Autodesk Inventor part; units mm, degrees
ref_plane "YZ Plane" through (0, 0, 0) normal (1, 0, 0) x (0, 1, 0)
ref_plane "XZ Plane" through (0, 0, 0) normal (0, 1, 0) x (-1, 0, 0)
ref_plane "XY Plane" through (0, 0, 0) normal (0, 0, 1) x (1, 0, 0)
sketch "Sketch1" plane through (0, 0, 0) normal (0, 0, 1) x (1, 0, 0)
  line L0 (10, 0) -> (10, 2)
  arc A0 (10, 2) -> (8.5, 3.5) centre (8.5, 2) ccw
  line L1 (8.5, 3.5) -> (-8.5, 3.5)
  arc A1 (-8.5, 3.5) -> (-10, 2) centre (-8.5, 2) ccw
  line L2 (-10, 2) -> (-8, 2)
  line L3 (-8, 2) -> (-8, 0)
  line L4 (-6, 0) -> (-8, 0)
  arc A2 (0, 0) -> (-6, 0) centre (-3, 0) ccw
  line L5 (7, 0) -> (0, 0)
  line L6 (7, 0) -> (7, 2.5)
  line L7 (7, 2.5) -> (9, 2.5)
  line L8 (9, 2.5) -> (9, 0)
  line L9 (10, 0) -> (9, 0)
  line L10 (-8, -2) -> (-10, -2)
  arc A3 (-10, -2) -> (-8.5, -3.5) centre (-8.5, -2) ccw
  line L11 (8.5, -3.5) -> (-8.5, -3.5)
  arc A4 (8.5, -3.5) -> (10, -2) centre (8.5, -2) ccw
  line L12 (10, 0) -> (10, -2)
  line L13 (9, 0) -> (10, 0)
  line L14 (9, 0) -> (9, -2.5)
  line L15 (9, -2.5) -> (7, -2.5)
  line L16 (7, -2.5) -> (7, 0)
  line L17 (0, 0) -> (7, 0)
  arc A5 (-6, 0) -> (0, 0) centre (-3, 0) ccw
  line L18 (-8, 0) -> (-6, 0)
  line L19 (-8, 0) -> (-8, -2)
  line L20 (-10, 2) -> (-10, 0)
  line L21 (-10, -2) -> (-10, 0)
  circle A6 centre (-8.5, 2) radius 1.25
  circle A7 centre (-8.5, -2) radius 1.25
  circle A8 centre (8.5, -2) radius 1.25
  circle A9 centre (8.5, 2) radius 1.25
  line L22 (8.5, 3.25) -> (-8.5, 3.25)
  line L23 (-9.75, 2) -> (-9.75, -2)
  line L24 (-8.5, -3.25) -> (8.5, -3.25)
  line L25 (9.75, 2) -> (9.75, -2)
  dimension "d22" = 0.25
extrude "Extrusion1" add sketch "Sketch1" along normal blind 2 contours L25 A8 L14 L9 | L9 L8 A9 L25 | L14 A8 L15 L16 L6 L7 A9 L8 | A9 L8 L7 | A8 L15 L14 | A9 L7 L8 | L14 L15 A8 | A9 L7 L6 L5 A2 L4 L3 A6 L22 | L24 A7 L19 L4 A5 L5 L16 L15 A8 | A6 L3 L2 | A7 L10 L19 | L2 L3 A6 | A6 L3 L19 A7 L23 | A7 L19 L10 | A5 A2
sketch "Sketch2" plane through (0, 0, 0) normal (0, 0, -1) x (-1, 0, 0)
  line L0 (-9, -2.5) -> (-7, -2.5)
  line L1 (-9, 2.5) -> (-9, 0)
  line L2 (-7, 2.5) -> (-9, 2.5)
  line L3 (-7, 0) -> (-7, 2.5)
  line L4 (-7, -2.5) -> (-7, 0)
  line L5 (-9, 0) -> (-9, -2.5)
  point P0 (0, 0)
extrude "Extrusion2" add sketch "Sketch2" along normal blind 4
sketch "Sketch3" plane through (0, 0, 0) normal (0, 0, -1) x (-1, 0, 0)
  line L0 (8, 2) -> (8, 0)
  line L1 (8, 0) -> (8, -2)
  line L2 (8, -2) -> (10, -2)
  line L3 (10, -2) -> (10, 0)
  line L4 (10, 2) -> (10, 0)
  line L5 (10, 2) -> (8, 2)
  line L6 (9.8, -1.8) -> (8.2, -1.8)
  line L7 (8.2, -1.8) -> (8.2, 1.8)
  line L8 (8.2, 1.8) -> (9.8, 1.8)
  line L9 (9.8, 1.8) -> (9.8, -1.8)
  point P0 (0, 0)
  dimension "d5" = 0.2
  dimension "d6" = 0.2
  dimension "d7" = 0.2
  dimension "d8" = 0.2
extrude "Extrusion3" add sketch "Sketch3" along normal blind 3.5 contours L6 L7 L8 L9
sketch "Sketch4" plane through (-9.8, -1.8, 0) normal (-1, 0, 0) x (0, 0, 1)
  line L0 (-3.5, 0) -> (-3.5, 3.6)
  line L1 (0, 3.6) -> (-3.5, 3.6)
  line L2 (0, 0) -> (-3.5, 0)
  line L3 (-3.5, 0) -> (-2, -1.2586)
  line L4 (-2, -1.2586) -> (-2, 5.3876)
  line L5 (-2, 5.3876) -> (-3.5, 3.6)
  point P0 (0, 1.8)
  dimension "d11" = 50
  dimension "d12" = 50
  dimension "d13" = 1.5
extrude "Extrusion4" add sketch "Sketch4" against normal up to surface (1.6 mm away)
fillet "Fillet2" radius 1 2 edges at (-9, -1.8, -3.5) (-9, 1.8, -3.5)
fillet "Fillet3" radius 0.5 2 edges at (-9, 3.5876, -2) (-9, -3.0586, -2)
fillet "Fillet4" radius 1 5 edges at (9.3839, 2.8839, 2) (9.75, 0, 2) (9.3839, -2.8839, 2) (0, -3.25, 2) (0, 3.25, 2)
sketch "Sketch7" plane through (0, 0, 2) normal (0, 0, 1) x (1, 0, 0)
  line L0 (-6.9276, 0) -> (0, 0) construction
  line L1 (-8, -1.2) -> (-3, -1.2)
  line L2 (-3, -1.2) -> (-3, -0.4)
  line L3 (-3, -0.4) -> (-8, -0.4)
  line L4 (-8, -0.4) -> (-8, -1.2)
  line L5 (-8, 1.2) -> (-7, 1.2)
  line L6 (-7, 1.2) -> (-7, 0.4)
  line L7 (-7, 0.4) -> (-8, 0.4)
  line L8 (-8, 0.4) -> (-8, 1.2)
  line L9 (-6, 0.4) -> (-6, 1.2)
  line L10 (-4, 1.2) -> (-3, 1.2)
  line L11 (-3, 1.2) -> (-3, 0.4)
  line L12 (-3, 0.4) -> (-4, 0.4)
  line L13 (-4, 0.4) -> (-4, 1.2)
  line L14 (-6, 1.2) -> (-5, 1.2)
  line L15 (-5, 1.2) -> (-5, 0.4)
  line L16 (-5, 0.4) -> (-6, 0.4)
  dimension "d31" = 5
  dimension "d32" = 0.8
  dimension "d33" = 0.4
  dimension "d35" = 0.8
  dimension "d36" = 1
  dimension "d37" = 1
  dimension "d38" = 1
  dimension "d39" = 1
  dimension "d40" = 1
  dimension "d41" = 3
  dimension "d42" = 0.4
extrude "Extrusion6" add sketch "Sketch7" along normal blind 0.5
sketch "Sketch8" plane through (0, 0, 2) normal (0, 0, 1) x (1, 0, 0)
  line L0 (-1, 1.5561) -> (6.4631, 1.5561) construction
  line L1 (6.4631, 1.5561) -> (6.4631, -1.5561) construction
  line L2 (6.4631, -1.5561) -> (-1, -1.5561) construction
  line L3 (-1, -1.5561) -> (-1, 1.5561) construction
  line L4 (1.4132, -1.5512) -> (-0.5999, -1.5512)
  line L5 (-0.5999, -1.5512) -> (-0.5999, -1.0201)
  line L6 (-0.5999, -1.0201) -> (0.0423, -1.0201)
  line L7 (0.0423, -1.0201) -> (0.0423, 0.5928)
  line L8 (0.0423, 0.5928) -> (-0.5999, 0.5928)
  line L9 (-0.5999, 0.5928) -> (-0.5999, 1.0893)
  spline S0 degree 2 poles (-0.5999, 1.0893) (-0.4591, 1.0893) (-0.18, 1.1263) (-0.096, 1.1658) knots 0 0 0 1 2 2 2
  spline S1 degree 2 poles (-0.096, 1.1658) (0.0004, 1.2152) (0.109, 1.3807) (0.1189, 1.5042) knots 0 0 0 1 2 2 2
  line L10 (0.1189, 1.5042) -> (0.7858, 1.5042)
  line L11 (0.7858, 1.5042) -> (0.7858, -1.0201)
  line L12 (0.7858, -1.0201) -> (1.4132, -1.0201)
  line L13 (1.4132, -1.0201) -> (1.4132, -1.5512)
  line L14 (4.2191, -1.5512) -> (1.9788, -1.5512)
  line L15 (1.9788, -1.5512) -> (1.9788, -1.0547)
  spline S2 degree 2 poles (1.9788, -1.0547) (2.2629, -0.8275) (2.7174, -0.4273) (2.8878, -0.247) knots 0 0 0 1 2 2 2
  spline S3 degree 2 poles (2.8878, -0.247) (3.1126, -0.0124) (3.3126, 0.3458) (3.3126, 0.5335) knots 0 0 0 1 2 2 2
  spline S4 degree 2 poles (3.3126, 0.5335) (3.3126, 0.7459) (3.0582, 0.9732) (2.831, 0.9732) knots 0 0 0 1 2 2 2
  spline S5 degree 2 poles (2.831, 0.9732) (2.7149, 0.9732) (2.5074, 0.9164) (2.4012, 0.8719) knots 0 0 0 1 2 2 2
  spline S6 degree 2 poles (2.4012, 0.8719) (2.2975, 0.825) (2.1493, 0.7262) (2.1122, 0.7015) knots 0 0 0 1 2 2 2
  line L16 (2.1122, 0.7015) -> (2.0529, 0.7015)
  line L17 (2.0529, 0.7015) -> (2.0529, 1.3659)
  spline S7 degree 2 poles (2.0529, 1.3659) (2.1814, 1.4277) (2.7297, 1.5561) (2.9841, 1.5561) knots 0 0 0 1 2 2 2
  spline S8 degree 2 poles (2.9841, 1.5561) (3.5275, 1.5561) (4.0858, 1.072) (4.0858, 0.6348) knots 0 0 0 1 2 2 2
  spline S9 degree 2 poles (4.0858, 0.6348) (4.0858, 0.3656) (3.8314, -0.1531) (3.5374, -0.4495) knots 0 0 0 1 2 2 2
  spline S10 degree 2 poles (3.5374, -0.4495) (3.3522, -0.6323) (3.0039, -0.9164) (2.9273, -0.9757) knots 0 0 0 1 2 2 2
  line L18 (2.9273, -0.9757) -> (4.2191, -0.9757)
  line L19 (4.2191, -0.9757) -> (4.2191, -1.5512)
  line L20 (7.2005, 1.4968) -> (6.1532, -1.5512)
  line L21 (6.1532, -1.5512) -> (5.3554, -1.5512)
  line L22 (5.3554, -1.5512) -> (4.3081, 1.4968)
  line L23 (4.3081, 1.4968) -> (5.1009, 1.4968)
  line L24 (5.1009, 1.4968) -> (5.7654, -0.5706)
  line L25 (5.7654, -0.5706) -> (6.4273, 1.4968)
  line L26 (6.4273, 1.4968) -> (7.2005, 1.4968)
  point P0 (0, 0)
  dimension "d45" = 3.1122
  dimension "d46" = 1.5561
  dimension "d47" = 1
extrude "Extrusion7" add sketch "Sketch8" along normal blind 0.5
equation "\"d6\" = d5"
equation "\"d7\" = d6"
equation "\"d8\" = d5"
equation "\"d12\" = d11"
equation "\"d33\" = 0.5 * d32"
equation "\"d35\" = d32"
equation "\"d36\" = 0.2 * d31"
equation "\"d37\" = d36"
equation "\"d38\" = d36"
equation "\"d39\" = d36"
equation "\"d40\" = d36"
equation "\"d42\" = d33"
properties part number "rubber-flippity-flap" material "Nylon 6/6"
Here's how the part is built. I have some questions about the finished solid (model axes, mm). A direction names the side the tool comes from. Give positions to 0.01 mm unless a question says otherwise; leave off trailing zeros. Loops run counter-clockwise (first coordinate to the right, second up) from the corner with the lowest first, then second, coordinate; pieces in that order, holes last. Notation, with made-up numbers: (46.5, 20.5) -> (96.5, 20.5) arc R14 ccw to (96.5, 35.5) -> close; hole circle Ø5 at (-36, -23.75). An arc over 180 degrees is marked (long way). Answer as a JSON object with one key per item and string values. Group by question number.
Item 1: Will these pins go through, and if not, where does the flat tip stop? pin 1 (2 mm diameter, centred on x = 0, z = -1.5, fed in from +Y); pin 2 (0.6 mm diameter, centred on y = 1, z = 2.5, fed in from +X); pin 3 (0.6 mm diameter, centred on y = 0.5, z = 2.5, fed in from +X); pin 4 (2 mm diameter, centred on x = -6, y = 1, fed in from -Z).
Item 2: Imagine slicing it at A-A on z = -2.5. Write out the boundary of the cut face in (x, y), then the cut area to 3 significant figures.
Item 3: On a 3-axis mill with a long thin cutter (end or side, diameter ignored), from which of +Z, -Z, +X, -X, +Y, -Y can I reach the whole of each face in a straight line? I mean faces 1 (the cylindrical face through (-9.394, 2.874, 0.493)), 2 (the flat face through (-9, -1.8, -1)), 3 (the flat face through (7, 0, -2)), 4 (the flat face through (4.84, -0.05, 2.25)), 5 (the flat face through (9, 0, -2)). Say none if no direction works.
Item 4: Imagine slicing it at B-B on x = -7.75. Write out the boundary of the cut face in (y, z).
Item 5: Thinking about a two-plate mould opening in X: for faces 6 (the flat face through (-0.12, 0.03, 2)), 7 (the flat face through (6.684, -0.006, 2.246)), 8 (the flat face through (5, 0, 2.5)), 9 (the flat face through (-9.8, 0, -2)), which applies, pulls with the +X half, pulls with the -X half, needs draft (parallel to the pull), parting line crosses it, or undercut?
Item 6: I need wall thicknesses on L1, parallel to X at y = 1.5, z = -3; L2, parallel to Z at x = 2.25, y = -0.5; L3, parallel to X at y = 2.25, z = -3.25. Which ranges of each line are inside material? Lowest first, please.
Item 7: Imagine slicing it at C-C on z = -0.75. Write out the boundary of the cut face in (x, y), then the cut area to 3 significant figures.
Item 8: Imagine slicing it at D-D on x = 4.5. Write out the boundary of the cut face in (y, z), then the cut area to 3 significant figures.
Answer list:
{
 "1": {"pin 1": "passes through", "pin 2": "stops at x = 7.13", "pin 3": "stops at x = 6.96", "pin 4": "stops at z = 0"},
 "2": {"outline": "(-9.8, -2.49) -> (-8.2, -2.49) -> (-8.2, 2.71) -> (-9.8, 2.71) -> close; (7, -2.5) -> (9, -2.5) -> (9, 2.5) -> (7, 2.5) -> close", "area": "18.3 mm2"},
 "3": {"face 1": "+Z, -X, +Y", "face 2": "-X, -Y", "face 3": "-Z, +Y, -Y", "face 4": "+Z, -Y", "face 5": "-Z, +X, +Y, -Y"},
 "4": {"outline": "(-3.25, 0) -> (3.25, 0) -> (3.25, 1) arc R1 ccw to (2.25, 2) -> (1.2, 2) -> (1.2, 2.5) -> (0.4, 2.5) -> (0.4, 2) -> (-0.4, 2) -> (-0.4, 2.5) -> (-1.2, 2.5) -> (-1.2, 2) -> (-2.25, 2) arc R1 ccw to (-3.25, 1) -> close"},
 "5": {"face 6": "undercut", "face 7": "pulls with the +X half", "face 8": "needs draft", "face 9": "pulls with the -X half"},
 "6": {"L1": "x = -9.8 to -8.2, 7 to 9", "L2": "z = 0 to 2", "L3": "x = 7 to 9"},
 "7": {"outline": "(-9.8, -1.8) -> (-8.2, -1.8) -> (-8.2, 1.8) -> (-9.8, 1.8) -> close; (7, -2.5) -> (9, -2.5) -> (9, 2.5) -> (7, 2.5) -> close", "area": "15.8 mm2"},
 "8": {"outline": "(-3.25, 0) -> (3.25, 0) -> (3.25, 1) arc R1 ccw to (2.25, 2) -> (1.5, 2) -> (1.5, 2.5) -> (0.94, 2.5) -> (0.94, 2) -> (-2.25, 2) arc R1 ccw to (-3.25, 1) -> close", "area": "12.9 mm2"}
}
